Geometry check sheet. Reference: the model listing, model coordinates, mm. Face numbers are marked on the shaded views. A direction names the side the tool comes from. Coordinates: 2 decimals unless noted, no trailing zeros. Loops run counter-clockwise (first coordinate to the right, second up) from the corner with the lowest first, then second, coordinate; pieces in that order, holes last. Notation, with made-up numbers: (35.5, 3) -> (41.5, 3) arc R20 ccw to (41.5, 35) -> close; hole circle Ø9 at (19.5, 13). An arc over 180 degrees is marked (long way). Answer as a JSON object with one key per item and string values.
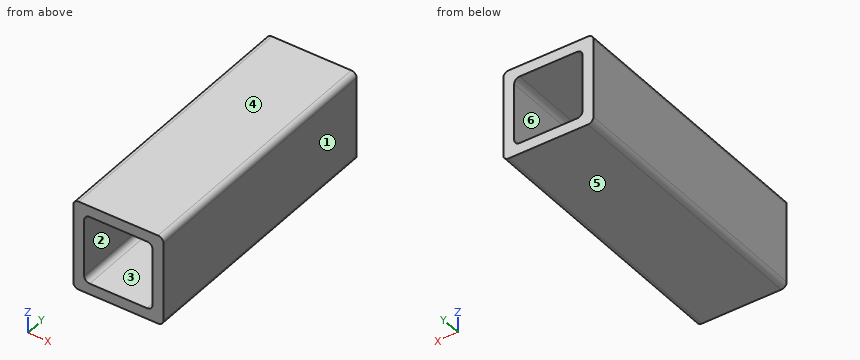
from build123d import *

# Parameters (mm, degrees)
CROQUIS1_W              = 16.5
CROQUIS1_H              = 16.5
CROQUIS1_W_2            = 12.5
CROQUIS1_H_2            = 12.5
SALIENTE_EXTRUIR1_DEPTH = 50
REDONDEO1_R             = 1


with BuildPart() as part:
    # Croquis1 → Saliente-Extruir1 (new body)
    with BuildSketch(Plane(origin=(0, 0, 0), x_dir=(1, 0, 0), z_dir=(0, 1, 0))):
        Rectangle(CROQUIS1_W, CROQUIS1_H)
        Rectangle(CROQUIS1_W_2, CROQUIS1_H_2, mode=Mode.SUBTRACT)
    extrude(amount=SALIENTE_EXTRUIR1_DEPTH)

    # Redondeo1
    redondeo1_edges = [part.edges().sort_by_distance(p)[0] for p in [
        (-6.25, 25, -6.25),
        (-6.25, 25, 6.25),
        (6.25, 25, 6.25),
        (6.25, 25, -6.25),
        (-8.25, 25, -8.25),
        (8.25, 25, -8.25),
        (8.25, 25, 8.25),
        (-8.25, 25, 8.25),
    ]]
    fillet(redondeo1_edges, radius=REDONDEO1_R)


solid = part.part
1. Depth check by flat-ended pin: P1, Ø5, axis at x = 2, z = -3.5, coming from the -Y side. Enter the tip coordinate at first touch or a pass-through.
Evaluation:
{"P1": "passes through"}
2. Section check A-A, the plane z = 1. Record the boundary of the cut face in (x, y).
Evaluation:
{"outline": "(-8.25, 0) -> (-6.25, 0) -> (-6.25, 50) -> (-8.25, 50) -> close; (6.25, 0) -> (8.25, 0) -> (8.25, 50) -> (6.25, 50) -> close"}
3. Tool access check on the marked faces 5 and 6. Record the directions out of +Z, -Z, +X, -X, +Y, -Y that give a thin tool (end or side, any length) a straight path to the whole face; none if there is none.
Evaluation:
{"face 5": "-Z, +X, -X, +Y, -Y", "face 6": "+Y, -Y"}
4. Mould release check, pull along X, two halves, no side actions. Record for the marked faces 1, 2, 3 and 4: released by +X, released by -X, zero draft, split by the parting line, or undercut.
Evaluation:
{"face 1": "released by +X", "face 2": "undercut", "face 3": "undercut", "face 4": "zero draft"}
5. Section check C-C, the plane y = 43. Record the boundary of the cut face in (x, z), then the cut area to 3 significant figures.
Evaluation:
{"outline": "(-8.25, -7.25) arc R1 ccw to (-7.25, -8.25) -> (7.25, -8.25) arc R1 ccw to (8.25, -7.25) -> (8.25, 7.25) arc R1 ccw to (7.25, 8.25) -> (-7.25, 8.25) arc R1 ccw to (-8.25, 7.25) -> close; hole (-6.25, -5.25) arc R1 ccw to (-5.25, -6.25) -> (5.25, -6.25) arc R1 ccw to (6.25, -5.25) -> (6.25, 5.25) arc R1 ccw to (5.25, 6.25) -> (-5.25, 6.25) arc R1 ccw to (-6.25, 5.25) -> close", "area": "116 mm^2"}
6. Thickness scan on probe 1 along Z at (x, y) = (-0.5, 42); probe 2 along X at (y, z) = (34.5, -6). Record the ranges inside material, lowest first. Write a range as from..to.
Evaluation:
{"probe 1": "z = -8.25..-6.25, 6.25..8.25", "probe 2": "x = -8.25..-5.91, 5.91..8.25"}
7. Section check B-B, the plane x = -2.25. Record the boundary of the cut face in (y, z), then the cut area to 3 significant figures.
Evaluation:
{"outline": "(0, -8.25) -> (50, -8.25) -> (50, -6.25) -> (0, -6.25) -> close; (0, 6.25) -> (50, 6.25) -> (50, 8.25) -> (0, 8.25) -> close", "area": "200 mm^2"}
